from build123d import *

# Parameters (mm, degrees)
F0_W     = 75
F0_H     = 120
F0_R     = 7.5
F1_DEPTH = 30
F2_R     = 5


with BuildPart() as f1:
    # F0 (on Front) → F1 (new body)
    with BuildSketch(Plane.XZ):
        with Locations((37.5, 60)):
            Rectangle(F0_W, F0_H)
        with Locations((37.5, 90)):
            Circle(F0_R, mode=Mode.SUBTRACT)
    extrude(amount=F1_DEPTH)

    # F2
    f2_edges = [f1.edges().sort_by_distance(p)[0] for p in [
        (37.5, -30, 120),
        (75, -15, 120),
        (37.5, 0, 120),
        (0, -15, 120),
        (0, 0, 60),
        (0, -30, 60),
        (75, 0, 60),
        (75, -30, 60),
        (37.5, -30, 0),
        (75, -15, 0),
        (37.5, 0, 0),
        (0, -15, 0),
    ]]
    fillet(f2_edges, radius=F2_R)


solid = f1.part
The model under review builds one solid part; all positions refer to its coordinate system, in mm. Coordinates: 2 decimals unless noted, no trailing zeros. Order: outer loops, then holes, each group sorted by start corner. A loop starts at its lowest first (then second) coordinate and runs counter-clockwise, first axis right, second up. Notation, with made-up numbers: (67.25, -10.75) -> (89.25, -10.75) arc R18 cw to (89.25, -3.75) -> close; hole circle Ø10 at (68, 11.5). An arc over 180 degrees is marked (long way). Answer in a Markdown table with one row per item.
(1) Consider section D-D (y = -26.25). Write out the cut boundary in (x, z), plus the area to 3 significant figures.
Answers:
| item | result |
|---|---|
| outline | (0.16, 5) arc R4.84 ccw to (5, 0.16) -> (70, 0.16) arc R4.84 ccw to (74.84, 5) -> (74.84, 115) arc R4.84 ccw to (70, 119.84) -> (5, 119.84) arc R4.84 ccw to (0.16, 115) -> close; hole circle Ø15 at (37.5, 90) |
| area | 8,740 mm² |
(2) Wall thickness on line 1 along Z through (x, y) = (37.5, -19.5); line 2 along Y through (x, z) = (4.5, 94); line 3 along X through (y, z) = (-4.5, 71): over which ranges is each line inside the solid? List them lowest first.
Answers:
| item | result |
|---|---|
| line 1 | 0 to 82.5, 97.5 to 120 |
| line 2 | -29.97 to -0.03 |
| line 3 | 0.03 to 74.97 |
(3) Consider section C-C (y = -7.25). Write out the cut boundary in (x, z), plus the area to 3 significant figures.
Answers:
| item | result |
|---|---|
| outline | (0, 5) arc R5 ccw to (5, 0) -> (70, 0) arc R5 ccw to (75, 5) -> (75, 115) arc R5 ccw to (70, 120) -> (5, 120) arc R5 ccw to (0, 115) -> close; hole circle Ø15 at (37.5, 90) |
| area | 8,800 mm² |
(4) Consider section B-B (z = 90). Write out the cut boundary in (x, y), plus the area to 3 significant figures.
Answers:
| item | result |
|---|---|
| outline | (0, -25) arc R5 ccw to (5, -30) -> (30, -30) -> (30, 0) -> (5, 0) arc R5 ccw to (0, -5) -> close; (45, -30) -> (70, -30) arc R5 ccw to (75, -25) -> (75, -5) arc R5 ccw to (70, 0) -> (45, 0) -> close |
| area | 1,780 mm² |
(5) Consider section A-A (x = 37.5). Write out the cut boundary in (y, z), plus the area to 3 significant figures.
Answers:
| item | result |
|---|---|
| outline | (-30, 5) arc R5 ccw to (-25, 0) -> (-5, 0) arc R5 ccw to (0, 5) -> (0, 82.5) -> (-30, 82.5) -> close; (-30, 97.5) -> (0, 97.5) -> (0, 115) arc R5 ccw to (-5, 120) -> (-25, 120) arc R5 ccw to (-30, 115) -> close |
| area | 3,130 mm² |
(6) The part is to be moulded in two halves that separate along X. For faces 1 (the cylindrical face through (1, -15, 118)), 2 (the flat face through (37, -15, 0)), 3 (the cylindrical face through (35.87, -14.79, 82.68)), 4 (the cylindrical face through (74, -28, 61)), say which applies: +X half, -X half, draft (parallel to the pull), parting line (faces both ways), or undercut.
Answers:
| item | result |
|---|---|
| face 1 | -X half |
| face 2 | draft |
| face 3 | undercut |
| face 4 | +X half |
